Build history of the part. All positions in model axes, mm. Face numbers are marked on the shaded views. A direction names the side the tool comes from. Round coordinates to 2 decimals unless told otherwise and drop trailing zeros. Write each loop counter-clockwise with the first axis right and the second up, starting at its lowest first coordinate (ties: lowest second). Pieces come first, ordered by that corner, then holes. Notation, with made-up numbers: (32.25, -27) -> (37.25, -27) arc R25 ccw to (37.25, -4) -> close; hole circle Ø11 at (18, 15.5). An arc over 180 degrees is marked (long way). Answer in a Markdown table with one row per item.
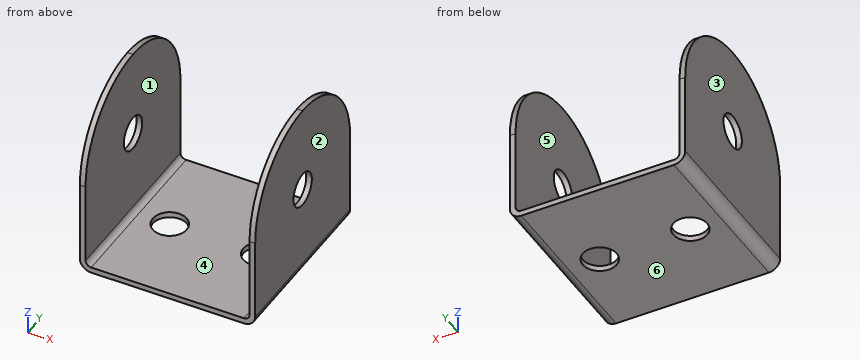
```python
from build123d import *

# Parameters (mm, degrees)
BRIDA_BASE1_DEPTH     = 15.5
CROQUIS5_R            = 1.5
CORTAR_EXTRUIR1_DEPTH = 29.789695
CROQUIS6_R            = 1.5
CORTAR_EXTRUIR2_DEPTH = 0.5


# Sheet-metal steps are written as plain solids
with BuildPart() as part:
    # Croquis1 → Brida base1 (new body)
    with BuildSketch(Plane(origin=(0, 0, 0), x_dir=(1, 0, 0), z_dir=(0, 1, 0))):
        with BuildLine():
            Line((-23.006869712, 2.664043993), (-23.006869712, 17.664043993))
            ThreePointArc((-23.006869712, 17.664043993), (-23.299762931, 18.371150774), (-24.006869712, 18.664043993))
            Line((-24.006869712, 18.664043993), (-37.506869712, 18.664043993))
            ThreePointArc((-37.506869712, 18.664043993), (-38.213976494, 18.371150774), (-38.506869712, 17.664043993))
            Line((-38.506869712, 17.664043993), (-38.506869712, 2.664043993))
            Line((-38.506869712, 2.664043993), (-38.006869712, 2.664043993))
            Line((-38.006869712, 2.664043993), (-38.006869712, 17.664043993))
            ThreePointArc((-38.006869712, 17.664043993), (-37.860423103, 18.017597384), (-37.506869712, 18.164043993))
            Line((-37.506869712, 18.164043993), (-24.006869712, 18.164043993))
            ThreePointArc((-24.006869712, 18.164043993), (-23.653316322, 18.017597384), (-23.506869712, 17.664043993))
            Line((-23.506869712, 17.664043993), (-23.506869712, 2.664043993))
            Line((-23.506869712, 2.664043993), (-23.006869712, 2.664043993))
        make_face()
    extrude(amount=BRIDA_BASE1_DEPTH)

    # Croquis5 → Cortar-Extruir1 (cut, through all)
    with BuildSketch(Plane(origin=(-23.006869712, 0, 0), x_dir=(0, 0, -1), z_dir=(1, 0, 0))):
        with BuildLine():
            ThreePointArc((2.664043993, 7.75), (4.933966439, 13.230077554), (10.414043993, 15.5))
            Line((10.414043993, 15.5), (2.664043993, 15.5))
            Line((2.664043993, 15.5), (2.664043993, 7.75))
        make_face()
        with BuildLine():
            ThreePointArc((10.414043993, 0), (4.933966439, 2.269922446), (2.664043993, 7.75))
            Line((2.664043993, 7.75), (2.664043993, 0))
            Line((2.664043993, 0), (10.414043993, 0))
        make_face()
        with Locations((10.414043993, 7.75)):
            Circle(CROQUIS5_R)
    extrude(amount=-CORTAR_EXTRUIR1_DEPTH, mode=Mode.SUBTRACT)

    # Croquis6 → Cortar-Extruir2 (cut)
    with BuildSketch(Plane.XY.offset(-18.164043993)):
        with Locations((-26.756869712, 7.75)):
            Circle(CROQUIS6_R)
        with Locations(Location((-34.756869712, 7.75, 0), (0, 0, 180))):
            Circle(CROQUIS6_R)
    extrude(amount=-CORTAR_EXTRUIR2_DEPTH, mode=Mode.SUBTRACT)


solid = part.part
```
Q1. Drop a flat-ended pin along its axis: P1, Ø4, axis at x = -32.5, y = 9.5, coming from the +Z side. Give the stop position or say it passes through.
A:
| item | result |
|---|---|
| P1 | z = -18.16 |
Q2. Wall check: line 1 (X direction, y = 14.5, z = -15.75); line 2 (Z direction, x = -30, y = 14.75). Give the ranges that are in metal, low to high. Write a range as [from, to].
A:
| item | result |
|---|---|
| line 1 | [-38.51, -38.01], [-23.51, -23.01] |
| line 2 | [-18.66, -18.16] |
Q3. Saw through at A-A on z = -4.75. Write the cut outline in (x, y), plus the area to 3 significant figures.
A:
| item | result |
|---|---|
| outline | (-38.51, 2.46) -> (-38.01, 2.46) -> (-38.01, 13.04) -> (-38.51, 13.04) -> close; (-23.51, 2.46) -> (-23.01, 2.46) -> (-23.01, 13.04) -> (-23.51, 13.04) -> close |
| area | 10.6 mm² |
Q4. Saw through at C-C on y = 11. Write the cut outline in (x, z).
A:
| item | result |
|---|---|
| outline | (-38.51, -17.66) arc R1 ccw to (-37.51, -18.66) -> (-24.01, -18.66) arc R1 ccw to (-23.01, -17.66) -> (-23.01, -3.38) -> (-23.51, -3.38) -> (-23.51, -17.66) arc R0.5 cw to (-24.01, -18.16) -> (-37.51, -18.16) arc R0.5 cw to (-38.01, -17.66) -> (-38.01, -3.38) -> (-38.51, -3.38) -> close |
Q5. Saw through at B-B on x = -34.5. Write the cut outline in (y, z).
A:
| item | result |
|---|---|
| outline | (0, -18.66) -> (6.27, -18.66) -> (6.27, -18.16) -> (0, -18.16) -> close; (9.23, -18.66) -> (15.5, -18.66) -> (15.5, -18.16) -> (9.23, -18.16) -> close |
Q6. Two-plate mould, pull along X, no slides. Class the marked faces 1, 2, 3 and 4: released by +X, released by -X, zero draft, split by the parting line, or undercut.
A:
| item | result |
|---|---|
| face 1 | undercut |
| face 2 | released by +X |
| face 3 | released by -X |
| face 4 | undercut |
Q7. Which spindle directions (+Z, -Z, +X, -X, +Y, -Y) get a long thin tool onto all of the face, cutting with end or side? Do the marked faces 5 and 6. Say none if no direction does.
A:
| item | result |
|---|---|
| face 5 | +Z, +Y, -Y |
| face 6 | -Z, +X, -X, +Y, -Y |
Q8. Saw through at D-D on x = -32.5. Write the cut outline in (y, z), plus the area to 3 significant figures.
A:
| item | result |
|---|---|
| outline | (0, -18.66) -> (15.5, -18.66) -> (15.5, -18.16) -> (0, -18.16) -> close |
| area | 7.75 mm² |
